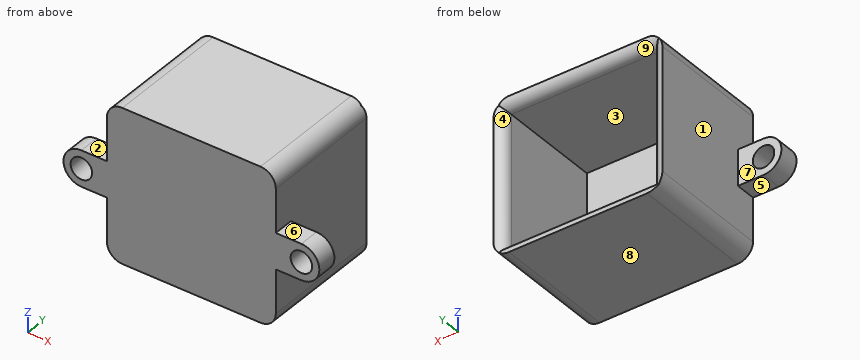
```python
from build123d import *

# Parameters (mm, degrees)
SKETCH2_W           = 33
SKETCH2_H           = 30
SKETCH2_W_2         = 29
SKETCH2_H_2         = 26
BOSS_EXTRUDE1_DEPTH = 22
SKETCH3_W           = 33
SKETCH3_H           = 30
BOSS_EXTRUDE2_DEPTH = 2
SKETCH4_R           = 2.1
BOSS_EXTRUDE3_DEPTH = 4
FILLET1_R           = 3
FILLET2_R           = 2


with BuildPart() as part:
    # Sketch2 → Boss-Extrude1 (new body)
    with BuildSketch(Plane(origin=(0, 0, 0), x_dir=(1, 0, 0), z_dir=(0, 1, 0))):
        Rectangle(SKETCH2_W, SKETCH2_H)
        Rectangle(SKETCH2_W_2, SKETCH2_H_2, mode=Mode.SUBTRACT)
    extrude(amount=BOSS_EXTRUDE1_DEPTH)

    # Sketch3 → Boss-Extrude2 (add)
    with BuildSketch(Plane.XZ):
        Rectangle(SKETCH3_W, SKETCH3_H)
    extrude(amount=BOSS_EXTRUDE2_DEPTH)

    # Sketch4 → Boss-Extrude3 (add)
    # profile 1 of 2: a face of its own
    with BuildSketch(Plane.XZ.offset(2)):
        with BuildLine():
            Line((-21.5, 3.5), (-16.5, 3.5))
            Line((-16.5, 3.5), (-16.5, -3.5))
            Line((-16.5, -3.5), (-21.5, -3.5))
            ThreePointArc((-21.5, -3.5), (-25, 0), (-21.5, 3.5))
        make_face()
        with Locations(Location((-21.5, 0, 0), (0, 0, 270))):
            Circle(SKETCH4_R, mode=Mode.SUBTRACT)
    # profile 2 of 2: a face of its own
    with BuildSketch(Plane.XZ.offset(2)):
        with BuildLine():
            Line((16.5, 3.5), (16.5, -3.5))
            Line((16.5, -3.5), (21.5, -3.5))
            ThreePointArc((21.5, -3.5), (25, 0), (21.5, 3.5))
            Line((21.5, 3.5), (16.5, 3.5))
        make_face()
        with Locations(Location((21.5, 0, 0), (0, 0, 90))):
            Circle(SKETCH4_R, mode=Mode.SUBTRACT)
    extrude(amount=-BOSS_EXTRUDE3_DEPTH)

    # Fillet1
    fillet1_edges = [part.edges().sort_by_distance(p)[0] for p in [
        (16.5, 10, 15),
        (-16.5, 10, 15),
        (-16.5, 10, -15),
        (16.5, 10, -15),
    ]]
    fillet(fillet1_edges, radius=FILLET1_R)

    # Fillet2
    # the kernel refuses this fillet: 2 mm, written as the material it takes off along each edge
    with BuildSketch(Plane(origin=(14.5, 22, -13), x_dir=(1, 0, 0), z_dir=(0, 0, 1)), Plane(origin=(-14.5, 22, 13), x_dir=(-1, 0, 0), z_dir=(0, 0, -1))) as fillet2_piece_1:
        with BuildLine():
            CenterArc((FILLET2_R, -FILLET2_R), FILLET2_R, 90, 90)
            Line((0, -FILLET2_R), (-FILLET2_R * 0.02, -FILLET2_R))
            Line((-FILLET2_R * 0.02, -FILLET2_R), (-FILLET2_R * 0.02, FILLET2_R * 0.02))
            Line((-FILLET2_R * 0.02, FILLET2_R * 0.02), (FILLET2_R, FILLET2_R * 0.02))
            Line((FILLET2_R, FILLET2_R * 0.02), (FILLET2_R, 0))
        make_face()
    extrude(amount=26, mode=Mode.SUBTRACT)
    with BuildSketch(Plane(origin=(-14.5, 22, -13), x_dir=(0, 0, -1), z_dir=(1, 0, 0)), Plane(origin=(14.5, 22, 13), x_dir=(0, 0, 1), z_dir=(-1, 0, 0))) as fillet2_piece_2:
        with BuildLine():
            CenterArc((FILLET2_R, -FILLET2_R), FILLET2_R, 90, 90)
            Line((0, -FILLET2_R), (-FILLET2_R * 0.02, -FILLET2_R))
            Line((-FILLET2_R * 0.02, -FILLET2_R), (-FILLET2_R * 0.02, FILLET2_R * 0.02))
            Line((-FILLET2_R * 0.02, FILLET2_R * 0.02), (FILLET2_R, FILLET2_R * 0.02))
            Line((FILLET2_R, FILLET2_R * 0.02), (FILLET2_R, 0))
        make_face()
    extrude(amount=29, mode=Mode.SUBTRACT)
    with BuildSketch(Plane(origin=(14.5, 22, -18), x_dir=(1, 0, 0), z_dir=(0, 0, 1))) as fillet2_piece_3a_section:
        with BuildLine():
            CenterArc((FILLET2_R, -FILLET2_R), FILLET2_R, 90, 90)
            Line((0, -FILLET2_R), (-FILLET2_R * 0.02, -FILLET2_R))
            Line((-FILLET2_R * 0.02, -FILLET2_R), (-FILLET2_R * 0.02, FILLET2_R * 0.02))
            Line((-FILLET2_R * 0.02, FILLET2_R * 0.02), (FILLET2_R, FILLET2_R * 0.02))
            Line((FILLET2_R, FILLET2_R * 0.02), (FILLET2_R, 0))
        make_face()
    fillet2_piece_3a = extrude(amount=31, mode=Mode.PRIVATE)
    fillet2_piece_3a = split(fillet2_piece_3a, bisect_by=Plane(origin=(14.952790229, 21.547209771, -13), z_dir=(0, 0, -1)), keep=Keep.TOP, mode=Mode.PRIVATE)
    with BuildSketch(Plane(origin=(-14.5, 22, -13), x_dir=(0, 0, -1), z_dir=(1, 0, 0))) as fillet2_piece_3b_section:
        with BuildLine():
            CenterArc((FILLET2_R, -FILLET2_R), FILLET2_R, 90, 90)
            Line((0, -FILLET2_R), (-FILLET2_R * 0.02, -FILLET2_R))
            Line((-FILLET2_R * 0.02, -FILLET2_R), (-FILLET2_R * 0.02, FILLET2_R * 0.02))
            Line((-FILLET2_R * 0.02, FILLET2_R * 0.02), (FILLET2_R, FILLET2_R * 0.02))
            Line((FILLET2_R, FILLET2_R * 0.02), (FILLET2_R, 0))
        make_face()
    fillet2_piece_3b = extrude(amount=34, mode=Mode.PRIVATE)
    fillet2_piece_3b = split(fillet2_piece_3b, bisect_by=Plane(origin=(14.5, 21.547209771, -13.452790229), z_dir=(1, 0, 0)), keep=Keep.TOP, mode=Mode.PRIVATE)
    fillet2_piece_3 = fillet2_piece_3a & fillet2_piece_3b
    add(fillet2_piece_3, mode=Mode.SUBTRACT)
    with BuildSketch(Plane(origin=(19.5, 22, 13), x_dir=(0, 0, 1), z_dir=(-1, 0, 0))) as fillet2_piece_4a_section:
        with BuildLine():
            CenterArc((FILLET2_R, -FILLET2_R), FILLET2_R, 90, 90)
            Line((0, -FILLET2_R), (-FILLET2_R * 0.02, -FILLET2_R))
            Line((-FILLET2_R * 0.02, -FILLET2_R), (-FILLET2_R * 0.02, FILLET2_R * 0.02))
            Line((-FILLET2_R * 0.02, FILLET2_R * 0.02), (FILLET2_R, FILLET2_R * 0.02))
            Line((FILLET2_R, FILLET2_R * 0.02), (FILLET2_R, 0))
        make_face()
    fillet2_piece_4a = extrude(amount=34, mode=Mode.PRIVATE)
    fillet2_piece_4a = split(fillet2_piece_4a, bisect_by=Plane(origin=(14.5, 21.547209771, 13.452790229), z_dir=(1, 0, 0)), keep=Keep.TOP, mode=Mode.PRIVATE)
    with BuildSketch(Plane(origin=(14.5, 22, -13), x_dir=(1, 0, 0), z_dir=(0, 0, 1))) as fillet2_piece_4b_section:
        with BuildLine():
            CenterArc((FILLET2_R, -FILLET2_R), FILLET2_R, 90, 90)
            Line((0, -FILLET2_R), (-FILLET2_R * 0.02, -FILLET2_R))
            Line((-FILLET2_R * 0.02, -FILLET2_R), (-FILLET2_R * 0.02, FILLET2_R * 0.02))
            Line((-FILLET2_R * 0.02, FILLET2_R * 0.02), (FILLET2_R, FILLET2_R * 0.02))
            Line((FILLET2_R, FILLET2_R * 0.02), (FILLET2_R, 0))
        make_face()
    fillet2_piece_4b = extrude(amount=31, mode=Mode.PRIVATE)
    fillet2_piece_4b = split(fillet2_piece_4b, bisect_by=Plane(origin=(14.952790229, 21.547209771, 13), z_dir=(0, 0, 1)), keep=Keep.TOP, mode=Mode.PRIVATE)
    fillet2_piece_4 = fillet2_piece_4a & fillet2_piece_4b
    add(fillet2_piece_4, mode=Mode.SUBTRACT)
    with BuildSketch(Plane(origin=(-14.5, 22, 13), x_dir=(-1, 0, 0), z_dir=(0, 0, -1))) as fillet2_piece_5a_section:
        with BuildLine():
            CenterArc((FILLET2_R, -FILLET2_R), FILLET2_R, 90, 90)
            Line((0, -FILLET2_R), (-FILLET2_R * 0.02, -FILLET2_R))
            Line((-FILLET2_R * 0.02, -FILLET2_R), (-FILLET2_R * 0.02, FILLET2_R * 0.02))
            Line((-FILLET2_R * 0.02, FILLET2_R * 0.02), (FILLET2_R, FILLET2_R * 0.02))
            Line((FILLET2_R, FILLET2_R * 0.02), (FILLET2_R, 0))
        make_face()
    fillet2_piece_5a = extrude(amount=31, mode=Mode.PRIVATE)
    fillet2_piece_5a = split(fillet2_piece_5a, bisect_by=Plane(origin=(-14.952790229, 21.547209771, -13), z_dir=(0, 0, -1)), keep=Keep.TOP, mode=Mode.PRIVATE)
    with BuildSketch(Plane(origin=(-19.5, 22, -13), x_dir=(0, 0, -1), z_dir=(1, 0, 0))) as fillet2_piece_5b_section:
        with BuildLine():
            CenterArc((FILLET2_R, -FILLET2_R), FILLET2_R, 90, 90)
            Line((0, -FILLET2_R), (-FILLET2_R * 0.02, -FILLET2_R))
            Line((-FILLET2_R * 0.02, -FILLET2_R), (-FILLET2_R * 0.02, FILLET2_R * 0.02))
            Line((-FILLET2_R * 0.02, FILLET2_R * 0.02), (FILLET2_R, FILLET2_R * 0.02))
            Line((FILLET2_R, FILLET2_R * 0.02), (FILLET2_R, 0))
        make_face()
    fillet2_piece_5b = extrude(amount=34, mode=Mode.PRIVATE)
    fillet2_piece_5b = split(fillet2_piece_5b, bisect_by=Plane(origin=(-14.5, 21.547209771, -13.452790229), z_dir=(-1, 0, 0)), keep=Keep.TOP, mode=Mode.PRIVATE)
    fillet2_piece_5 = fillet2_piece_5a & fillet2_piece_5b
    add(fillet2_piece_5, mode=Mode.SUBTRACT)
    with BuildSketch(Plane(origin=(-14.5, 22, 18), x_dir=(-1, 0, 0), z_dir=(0, 0, -1))) as fillet2_piece_6a_section:
        with BuildLine():
            CenterArc((FILLET2_R, -FILLET2_R), FILLET2_R, 90, 90)
            Line((0, -FILLET2_R), (-FILLET2_R * 0.02, -FILLET2_R))
            Line((-FILLET2_R * 0.02, -FILLET2_R), (-FILLET2_R * 0.02, FILLET2_R * 0.02))
            Line((-FILLET2_R * 0.02, FILLET2_R * 0.02), (FILLET2_R, FILLET2_R * 0.02))
            Line((FILLET2_R, FILLET2_R * 0.02), (FILLET2_R, 0))
        make_face()
    fillet2_piece_6a = extrude(amount=31, mode=Mode.PRIVATE)
    fillet2_piece_6a = split(fillet2_piece_6a, bisect_by=Plane(origin=(-14.952790229, 21.547209771, 13), z_dir=(0, 0, 1)), keep=Keep.TOP, mode=Mode.PRIVATE)
    with BuildSketch(Plane(origin=(14.5, 22, 13), x_dir=(0, 0, 1), z_dir=(-1, 0, 0))) as fillet2_piece_6b_section:
        with BuildLine():
            CenterArc((FILLET2_R, -FILLET2_R), FILLET2_R, 90, 90)
            Line((0, -FILLET2_R), (-FILLET2_R * 0.02, -FILLET2_R))
            Line((-FILLET2_R * 0.02, -FILLET2_R), (-FILLET2_R * 0.02, FILLET2_R * 0.02))
            Line((-FILLET2_R * 0.02, FILLET2_R * 0.02), (FILLET2_R, FILLET2_R * 0.02))
            Line((FILLET2_R, FILLET2_R * 0.02), (FILLET2_R, 0))
        make_face()
    fillet2_piece_6b = extrude(amount=34, mode=Mode.PRIVATE)
    fillet2_piece_6b = split(fillet2_piece_6b, bisect_by=Plane(origin=(-14.5, 21.547209771, 13.452790229), z_dir=(-1, 0, 0)), keep=Keep.TOP, mode=Mode.PRIVATE)
    fillet2_piece_6 = fillet2_piece_6a & fillet2_piece_6b
    add(fillet2_piece_6, mode=Mode.SUBTRACT)


solid = part.part
```
Input: part model. Units: mm. Frame: model coordinates. Face numbers are marked on the shaded views. A direction names the side the tool comes from. Give positions to 0.01 mm unless a question says otherwise; leave off trailing zeros. Order: outer loops, then holes, each group sorted by start corner. A loop starts at its lowest first (then second) coordinate and runs counter-clockwise, first axis right, second up. Notation, with made-up numbers: (32, -20) - (89, -20) arc R7 cw to (89, -13) - close; hole circle Ø9 at (47.5, -16.5). An arc over 180 degrees is marked (long way). Use a Markdown table: item, result.
(1) Section query D-D (z = 10). Output: boundary loops of the cut face in (x, y), then the cut area to 3 significant figures.
Computed values:
| item | result |
|---|---|
| outline | (-16.5, -2) - (16.5, -2) - (16.5, 22) arc R2 ccw to (14.5, 20) - (14.5, 0) - (-14.5, 0) - (-14.5, 20) arc R2 ccw to (-16.5, 22) - close |
| area | 152 mm2 |
(2) Section query A-A (y = 5.5). Output: boundary loops of the cut face in (x, z).
Computed values:
| item | result |
|---|---|
| outline | (-16.5, -12) arc R3 ccw to (-13.5, -15) - (13.5, -15) arc R3 ccw to (16.5, -12) - (16.5, 12) arc R3 ccw to (13.5, 15) - (-13.5, 15) arc R3 ccw to (-16.5, 12) - close; hole (-14.5, -13) - (14.5, -13) - (14.5, 13) - (-14.5, 13) - close |
(3) Pin query (flat end, axial travel): pin 1 (6.5 mm diameter, centred on x = -21.5, z = 0, fed in from +Y); pin 2 (12 mm diameter, centred on y = 9, z = -3.5, fed in from +X); pin 3 (4.5 mm diameter, centred on x = -18, y = -0.5, fed in from -Z). Return the tip coordinate at first contact, or that it passes through.
Computed values:
| item | result |
|---|---|
| pin 1 | stops at y = 2 |
| pin 2 | stops at x = 16.5 |
| pin 3 | stops at z = -13.98 |
(4) Section query C-C (x = 3). Output: boundary loops of the cut face in (y, z), then the cut area to 3 significant figures.
Computed values:
| item | result |
|---|---|
| outline | (-2, -15) - (22, -15) arc R2 ccw to (20, -13) - (0, -13) - (0, 13) - (20, 13) arc R2 ccw to (22, 15) - (-2, 15) - close |
| area | 146 mm2 |
(5) Section query B-B (z = 0). Output: boundary loops of the cut face in (x, y), then the cut area to 3 significant figures.
Computed values:
| item | result |
|---|---|
| outline | (-25, -2) - (-23.6, -2) - (-23.6, 2) - (-25, 2) - close; (-19.4, -2) - (19.4, -2) - (19.4, 2) - (16.5, 2) - (16.5, 22) arc R2 ccw to (14.5, 20) - (14.5, 0) - (-14.5, 0) - (-14.5, 20) arc R2 ccw to (-16.5, 22) - (-16.5, 2) - (-19.4, 2) - close; (23.6, -2) - (25, -2) - (25, 2) - (23.6, 2) - close |
| area | 187 mm2 |
(6) Access query for the marked faces 5, 6, 7, 8 and 9. Directions: +Z, -Z, +X, -X, +Y, -Y. A direction counts if a zero-diameter tool reaches every point of the face in a straight line with its end or side. Return the directions, or none.
Computed values:
| item | result |
|---|---|
| face 5 | -Z, -X, +Y, -Y |
| face 6 | +Z, +X, +Y, -Y |
| face 7 | +Z, -Z, -X, +Y |
| face 8 | -Z, +X, -X, +Y, -Y |
| face 9 | +Y |
(7) Line query: line 1 (X direction, y = 0.95, z = 0); line 2 (X direction, y = -0.75, z = 0); line 3 (Z direction, x = 21.5, y = 1). Output: solid intervals per line, ascending. Write a range as from..to.
Computed values:
| item | result |
|---|---|
| line 1 | x = -25..-23.6, -19.4..-14.5, 14.5..19.4, 23.6..25 |
| line 2 | x = -25..-23.6, -19.4..19.4, 23.6..25 |
| line 3 | z = -3.5..-2.1, 2.1..3.5 |
(8) Draft query along Z for the marked faces 1, 2, 3 and 4. Return one class per face: released by +Z, released by -Z, zero draft, split by the parting line, or undercut.
Computed values:
| item | result |
|---|---|
| face 1 | zero draft |
| face 2 | released by +Z |
| face 3 | undercut |
| face 4 | undercut |
